Build history of the part. All positions in model axes, mm. Face numbers are marked on the shaded views. A direction names the side the tool comes from. Coordinates: 2 decimals unless noted, no trailing zeros. Write each loop counter-clockwise with the first axis right and the second up, starting at its lowest first coordinate (ties: lowest second). Pieces come first, ordered by that corner, then holes.
```python
from build123d import *

# Parameters (mm, degrees)
SKETCH1_R           = 1.2
BOSS_EXTRUDE1_DEPTH = 2
SKETCH2_W           = 2
SKETCH2_H           = 8
BOSS_EXTRUDE2_DEPTH = 1.25
SKETCH3_W           = 2
SKETCH3_H           = 8
BOSS_EXTRUDE3_DEPTH = 2.25
CUT_EXTRUDE1_DEPTH  = 1
CUT_EXTRUDE2_DEPTH  = 2.1
CUT_EXTRUDE3_DEPTH  = 2.1
CHAMFER1_SIZE       = 1.5
CHAMFER2_SIZE       = 0.5


with BuildPart() as part:
    # Sketch1 → Boss-Extrude1 (new body)
    with BuildSketch(Plane(origin=(0, 0, 0), x_dir=(1, 0, 0), z_dir=(0, 1, 0))):
        Polygon((-8.6, -10.1), (9.5, -10.1), (9.5, -4), (11.6, -4), (11.6, 4), (9.5, 4), (9.5, 10.1), (-8.6, 10.1), (-8.6, 4), (-7.95, 4), (-7.95, 1.9), (-1.6, 1.9), (-1.6, -1.9), (-7.95, -1.9), (-7.95, -4), (-8.6, -4), align=None)
        with Locations(Location((0, 0, 0), (0, 0, 270))):
            Circle(SKETCH1_R, mode=Mode.SUBTRACT)
    extrude(amount=BOSS_EXTRUDE1_DEPTH)

    # Sketch2 → Boss-Extrude2 (add)
    with BuildSketch(Plane(origin=(0, 2, 0), x_dir=(1, 0, 0), z_dir=(0, 1, 0))):
        Polygon((-8.6, -4), (-7.95, -4), (-7.95, -1.9), (-2.5, -1.9), (-2.5, -4), (-6.6, -4), (-6.6, -8.1), (3.7, -8.1), (5.7, -10.1), (-8.6, -10.1), align=None)
        Polygon((-8.6, 10.1), (-8.6, 4), (-7.95, 4), (-7.95, 1.9), (-2.5, 1.9), (-2.5, 4), (-6.6, 4), (-6.6, 8.1), (3.7, 8.1), (5.7, 10.1), align=None)
        with Locations((10.6, 0)):
            Rectangle(SKETCH2_W, SKETCH2_H)
    extrude(amount=BOSS_EXTRUDE2_DEPTH)

    # Sketch3 → Boss-Extrude3 (add)
    with BuildSketch(Plane(origin=(0, 3.25, 0), x_dir=(1, 0, 0), z_dir=(0, 1, 0))):
        with Locations((10.6, 0)):
            Rectangle(SKETCH3_W, SKETCH3_H)
        Polygon((3.7, -8.1), (-6, -8.1), (-6, -10.1), (5.7, -10.1), align=None)
        Polygon((3.7, 8.1), (-6, 8.1), (-6, 10.1), (4.55, 10.1), (4.55, 8.95), align=None)
    extrude(amount=BOSS_EXTRUDE3_DEPTH)

    # Sketch4 → Cut-Extrude1 (cut)
    with BuildSketch(Plane.XZ):
        Polygon((-2.309401077, 0), (-1.154700538, -2), (1.154700538, -2), (2.309401077, 0), (1.154700538, 2), (-1.154700538, 2), align=None)
    extrude(amount=-CUT_EXTRUDE1_DEPTH, mode=Mode.SUBTRACT)

    # Sketch5 → Cut-Extrude2 (cut)
    with BuildSketch(Plane(origin=(0, 0, 1.9), x_dir=(-1, 0, 0), z_dir=(0, 0, -1))):
        Polygon((7.95, 0.75), (5.45, 0.75), (2.95, 3.25), (7.95, 3.25), align=None)
    extrude(amount=-CUT_EXTRUDE2_DEPTH, mode=Mode.SUBTRACT)

    # Sketch6 → Cut-Extrude3 (cut)
    with BuildSketch(Plane.XY.offset(-1.9)):
        Polygon((-7.95, 3.25), (-7.95, 0.75), (-5.45, 0.75), (-2.95, 3.25), align=None)
    extrude(amount=-CUT_EXTRUDE3_DEPTH, mode=Mode.SUBTRACT)

    # Chamfer1
    chamfer1_edges = [part.edges().sort_by_distance(p)[0] for p in [
        (-8.6, 1.625, -10.1),
        (-8.6, 1.625, 10.1),
    ]]
    chamfer(chamfer1_edges, length=CHAMFER1_SIZE)

    # Chamfer2
    chamfer2_edges = [part.edges().sort_by_distance(p)[0] for p in [
        (11.6, 2.75, -4),
        (11.6, 2.75, 4),
        (-8.6, 0, 6.3),
        (-7.85, 0, 9.35),
        (-8.6, 0, -6.3),
        (-7.85, 0, -9.35),
        (1.2, 0, -10.1),
        (9.5, 0, -7.05),
        (10.55, 0, -4),
        (1.2, 0, 10.1),
        (9.5, 0, 7.05),
        (10.55, 0, 4),
        (11.6, 0, 0),
        (-1.377350269, 0, -1.614359354),
        (0, 0, -2),
        (-1.377350269, 0, 1.614359354),
        (0, 0, 2),
        (1.732050808, 0, 1),
        (1.732050808, 0, -1),
        (-1.15, 5.5, -8.1),
        (-6, 4.375, -8.1),
        (-6.3, 3.25, -8.1),
        (-6.6, 3.25, -6.05),
        (-7.6, 3.25, -4),
        (-6.55, 3.25, -10.1),
        (-7.85, 3.25, -9.35),
        (-8.6, 3.25, -6.3),
        (-7.95, 0.75, 2.95),
        (-7.95, 0.75, -2.95),
        (9.6, 3.75, 4),
        (9.6, 3.75, -4),
        (9.6, 5.5, 0),
        (-1.15, 5.5, 8.1),
        (-6, 4.375, 8.1),
        (-6.3, 3.25, 8.1),
        (-6.6, 3.25, 6.05),
        (-7.6, 3.25, 4),
        (-6.55, 3.25, 10.1),
        (-7.85, 3.25, 9.35),
        (-8.6, 3.25, 6.3),
        (9.5, 1, -10.1),
        (9.5, 1, 10.1),
        (4.125, 5.5, -8.525),
        (4.7, 5.5, 9.1),
        (-6, 4.375, -10.1),
        (-6, 4.375, 10.1),
    ]]
    chamfer(chamfer2_edges, length=CHAMFER2_SIZE)


solid = part.part
```
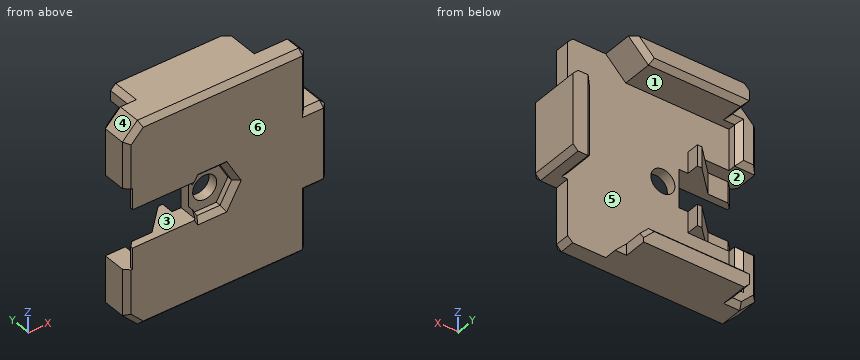
1. Flat gauge pins, fed straight in: pin 1 (6 mm diameter, centred on x = 9.5, z = -6.5, fed in from -Y); pin 2 (1.2 mm diameter, centred on y = 1, z = -6, fed in from +X); pin 3 (1.5 mm diameter, centred on x = -6, z = 0, fed in from +Y); pin 4 (0.9 mm diameter, centred on y = 4, z = 0, fed in from -X). Where does each tip first touch, or does it go through?
Computed values:
pin 1: stops at y = 0
pin 2: stops at x = 9.5
pin 3: passes through
pin 4: stops at x = 9.6
2. Probe line 1 along X through (y, z) = (1.8, 0); line 2 along Z through (x, y) = (2.5, 3.8); line 3 along Z through (x, y) = (0, 1.35). List the from-to ranges inside material, lowest first.
Computed values:
line 1: x = -1.6 to -1.2, 1.2 to 11.6
line 2: z = -10.1 to -8.1, 8.1 to 10.1
line 3: z = -10.1 to -1.2, 1.2 to 10.1
3. 3-axis set-ups, long thin cutter, end or side, ignore diameter. For the marked faces 1, 2 and 3: which of +Z, -Z, +X, -X, +Y, -Y reach the whole face in a straight line?
Computed values:
face 1: +X, +Y
face 2: -X, +Y
face 3: -X, +Y, -Y
4. Mould opens along X. For the marked faces 4, 5 and 6 say: +X half, -X half, draft (parallel to the pull), parting line (faces both ways), or undercut.
Computed values:
face 4: -X half
face 5: undercut
face 6: draft
5. Saw through at A-A on x = 0. List the corners of the cut face in (y, z), plus the area to 4 significant figures.
Computed values:
outline: (0, -9.6) - (0.5, -10.1) - (5.5, -10.1) - (5.5, -8.6) - (5, -8.1) - (2, -8.1) - (2, -1.2) - (1, -1.2) - (1, -2) - (0.5, -2) - (0, -2.5) - close; (0, 2.5) - (0.5, 2) - (1, 2) - (1, 1.2) - (2, 1.2) - (2, 8.1) - (5, 8.1) - (5.5, 8.6) - (5.5, 10.1) - (0.5, 10.1) - (0, 9.6) - close
area: 47.25 mm2
6. Saw through at B-B on z = -6.75. List the corners of the cut face in (x, y), plus the area to 3 significant figures.
Computed values:
outline: (-8.6, 0.5) - (-8.1, 0) - (9, 0) - (9.5, 0.5) - (9.5, 2) - (-6.6, 2) - (-6.6, 2.75) - (-7.1, 3.25) - (-8.1, 3.25) - (-8.6, 2.75) - close
area: 38.2 mm2
